Check sheet for the modelled part. Datum: model origin and axes. Units: mm. Round coordinates to 2 decimals unless told otherwise and drop trailing zeros. Write each loop counter-clockwise with the first axis right and the second up, starting at its lowest first coordinate (ties: lowest second). Pieces come first, ordered by that corner, then holes. Notation, with made-up numbers: (19, 20.25) -> (60, 20.25) arc R20 ccw to (60, 36.25) -> close; hole circle Ø8 at (-18, -33). An arc over 180 degrees is marked (long way). One line per item, written item: value.
Autodesk Inventor part; units mm, degrees
ref_plane "Work Plane1" through (25, 0, 0) normal (1, 0, 0) x (0, 1, 0)
ref_plane "XZ Plane" through (0, 0, 0) normal (0, 1, 0) x (-1, 0, 0)
ref_plane "XY Plane" through (0, 0, 0) normal (0, 0, 1) x (1, 0, 0)
sketch "Sketch1" plane through (0, 0, 0) normal (0, 0, 1) x (1, 0, 0)
  circle A0 centre (0, 0) radius 25
  dimension "d0" = 50
extrude "Extrusion1" add sketch "Sketch1" along normal mid plane 10
ref_plane "Work Plane1" through (25, 0, 0) normal (1, 0, 0) x (0, 1, 0)
sketch "Sketch2" plane through (25, 0, 0) normal (1, 0, 0) x (0, 1, 0)
  circle A0 centre (0, 0) radius 5
  line L0 (-25, -5) -> (25, -5)
  point P0 (0, 0)
extrude "Extrusion2" add sketch "Sketch2" along normal mid plane 2
sketch "Sketch3" plane through (26, 0, 0) normal (1, 0, 0) x (0, 0, -1)
  circle A0 centre (0, 0) radius 3.5
  point P0 (0, 0)
  dimension "d5" = 7
extrude "Extrusion3" add sketch "Sketch3" along normal blind 1
chamfer "Chamfer1" distance 1 angle 45 1 edges at (26, 0, 3.5)
pattern_circular "Circular Pattern1" count 3 over 360 about axis through (0, 0, 0) along (0, 0, 1) of "Extrusion2", "Extrusion3", "Chamfer1"
properties part number "Platform"
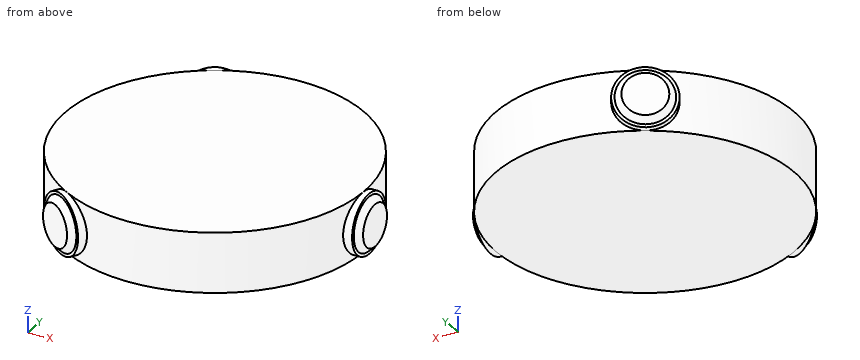
Item 1: Sectioned sample at B-B on y = -16. Enter the section's corners in (x, z), and give its area (3 significant figures).
Answer:
outline: (-19.21, -5) -> (19.21, -5) -> (19.21, 5) -> (-19.21, 5) -> close
area: 384 mm^2
Item 2: Thickness scan on line 1 (X direction, y = -12.5, z = 1); line 2 (Y direction, x = -13.5, z = -1.75); line 3 (Y direction, x = -10, z = 2.25). Record the ranges inside material, lowest first.
Answer:
line 1: x = -21.65 to 21.65
line 2: y = -23.38 to 23.38
line 3: y = -24.54 to 24.54
Item 3: Depth check by flat-ended pin: P1, Ø1, axis at x = 11, z = 3.5, coming from the +Y side; P2, Ø1.5, axis at x = 21.5, z = 0, coming from the -Y side; P3, Ø5, axis at x = -1.5, z = 2, coming from the -Y side. Enter the tip coordinate at first touch or a pass-through.
Answer:
P1: stops at y = 22.69
P2: stops at y = -13.94
P3: stops at y = -25
